Check sheet for the modelled part. Datum: model origin and axes. Units: mm. Face numbers are marked on the shaded views. A direction names the side the tool comes from. Round coordinates to 2 decimals unless told otherwise and drop trailing zeros. Order: outer loops, then holes, each group sorted by start corner. A loop starts at its lowest first (then second) coordinate and runs counter-clockwise, first axis right, second up.
Q1. Depth check by flat-ended pin: P1, Ø6, axis at x = 14.5, z = 18.5, coming from the -Y side. Enter the tip coordinate at first touch or a pass-through.
Q2. Set-up check for the marked faces 1 and 2: record each of +Z, -Z, +X, -X, +Y, -Y from which the full face is reachable in a straight line by a thin tool's end or side.
Q3. Scan lines: probe 1 along Z at (x, y) = (37, -17); probe 2 along Z at (x, y) = (-12.5, -27.5); probe 3 along X at (y, z) = (-14, -15). Record each from-to range of solid material in increasing order.
Q4. Mould release check, pull along Z, two halves, no side actions. Record for the marked faces 3, 4 and 5: +Z half, -Z half, draft (parallel to the pull), parting line (faces both ways), or undercut.
Q5. Cross-section at B-B on x = -82. Record the cut outline in (y, z).
Q6. Cross-section at C-C on z = 17. Record the cut outline in (x, y).
Q7. Cross-section at D-D on x = 0.5. Record the cut outline in (y, z).
Q8. Cross-section at A-A on z = -12. Record the cut outline in (x, y), then the cut area to 3 significant figures.
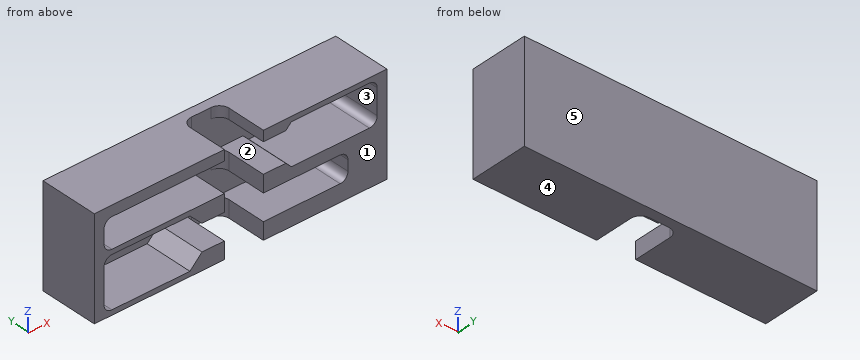
from build123d import *

# Parameters (mm, degrees)
F0_W          = 190.5
F0_H          = 65.278
F1_DEPTH      = 31.75
F1_DEPTH_BACK = 6.35
F3_DEPTH      = 31.75
F4_R          = 5.08
F5_W          = 25.4
F5_H          = 65.278
F6_DEPTH      = 31.75
F7_R          = 6.35


with BuildPart() as f1:
    # F0 (on Front) → F1 (new body, two sides)
    with BuildSketch(Plane.XZ) as f1_sk:
        Rectangle(F0_W, F0_H)
    extrude(amount=F1_DEPTH)
    extrude(f1_sk.sketch, amount=-F1_DEPTH_BACK)

    # F2 (on Front) → F3 (cut, through all)
    with BuildSketch(Plane.XZ):
        Polygon((29.337, 25.781), (-88.9, 25.781), (-88.9, 6.477), (29.337, 6.477), (33.02, 2.794), (88.9, 2.794), (88.9, 29.464), (33.02, 29.464), align=None)
        Polygon((-33.02, 3.302), (-88.9, 3.302), (-88.9, -29.464), (-33.02, -29.464), (-25.146, -21.59), (69.85, -21.59), (69.85, -4.572), (-25.146, -4.572), align=None)
    extrude(amount=F3_DEPTH, mode=Mode.SUBTRACT)

    # F4
    f4_edges = [f1.edges().sort_by_distance(p)[0] for p in [
        (-88.9, -15.875, 3.302),
        (-88.9, -15.875, -29.464),
        (69.85, -15.875, -4.572),
        (69.85, -15.875, -21.59),
        (88.9, -15.875, 2.794),
        (88.9, -15.875, 29.464),
        (-88.9, -15.875, 25.781),
        (-88.9, -15.875, 6.477),
    ]]
    fillet(f4_edges, radius=F4_R)

    # F5 (on face) → F6 (cut)
    with BuildSketch(Plane.XZ.offset(31.75)):
        with Locations((2.0955, 0)):
            Rectangle(F5_W, F5_H)
    extrude(amount=-F6_DEPTH, mode=Mode.SUBTRACT)

    # F7
    f7_edges = [f1.edges().sort_by_distance(p)[0] for p in [
        (14.7955, 0, -27.1145),
        (14.7955, 0, 0.9525),
        (14.7955, 0, 29.21),
        (-10.6045, 0, 29.21),
        (-10.6045, 0, 0.9525),
        (-10.6045, 0, -27.1145),
    ]]
    fillet(f7_edges, radius=F7_R)


solid = f1.part
Results found:
1. P1: stops at y = 0
2. face 1: +Z, -Z, +X, -X, -Y
2. face 2: -Y
3. probe 1: z = -32.64 to -21.59, -4.57 to 2.79, 29.46 to 32.64
3. probe 2: z = -32.64 to -21.59, -4.57 to 6.48, 25.78 to 32.64
3. probe 3: x = -95.25 to -88.9, 69.85 to 95.25
4. face 3: undercut
4. face 4: -Z half
4. face 5: draft
5. outline: (-31.75, -32.64) - (6.35, -32.64) - (6.35, 32.64) - (-31.75, 32.64) - (-31.75, 25.78) - (0, 25.78) - (0, 6.48) - (-31.75, 6.48) - (-31.75, 3.3) - (0, 3.3) - (0, -29.46) - (-31.75, -29.46) - close
6. outline: (-95.25, -31.75) - (-88.9, -31.75) - (-88.9, 0) - (88.9, 0) - (88.9, -31.75) - (95.25, -31.75) - (95.25, 6.35) - (-95.25, 6.35) - close
7. outline: (0, -32.64) - (6.35, -32.64) - (6.35, 32.64) - (0, 32.64) - close
8. outline: (-95.25, -31.75) - (-88.9, -31.75) - (-88.9, 0) - (69.85, 0) - (69.85, -31.75) - (95.25, -31.75) - (95.25, 6.35) - (-95.25, 6.35) - close
8. area: 2,220 mm2
